The drawing under review shows one solid part. Ordinate dimensions are in mm from its lowest x, y, z. A direction names the side the tool comes from. Round coordinates to 2 decimals unless told otherwise and drop trailing zeros. Write each loop counter-clockwise with the first axis right and the second up, starting at its lowest first coordinate (ties: lowest second). Pieces come first, ordered by that corner, then holes. Notation, with made-up numbers: (-37.5, 71) - (-15.5, 71) arc R22 ccw to (-15.5, 80) - close; hole circle Ø4 at (76, 27.5). An arc over 180 degrees is marked (long way). One line per question, with ' | ' between items. Start each with the question number.
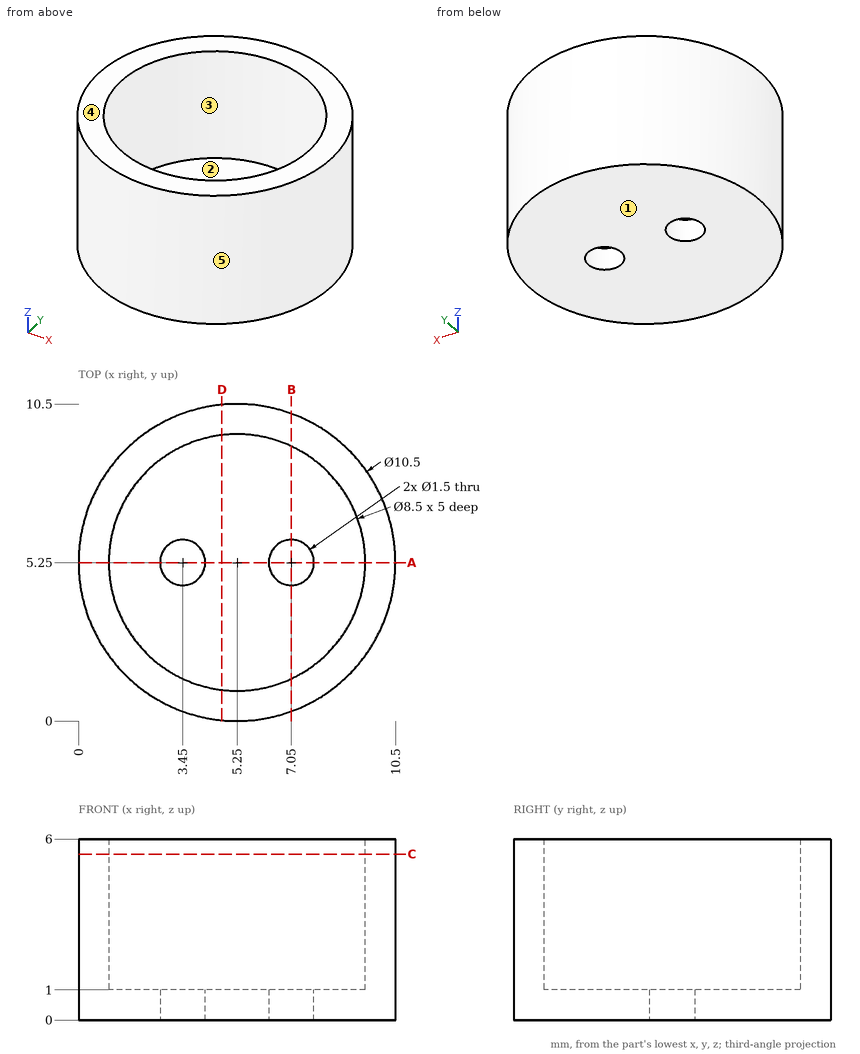
1. Add section B-B, the plane x = 7.05. Write out the cut boundary in (y, z).
2. The part is to be moulded in two halves that separate along Y. For the marked faces 3, 4 and 5, say which applies: pulls with the +Y half, pulls with the -Y half, needs draft (parallel to the pull), parting line crosses it, or undercut.
3. Machinability: for the marked faces 1 and 2, which of the approach directions +Z, -Z, +X, -X, +Y, -Y give a long, thin tool a straight path to every point of the face, cutting with its end or side? Answer none if there is none.
4. Clearance check with flat-ended pins moving along their axes: P1, Ø1.7, axis at x = 7.05, y = 5.25, coming from the +Z side; P2, Ø1.5, axis at x = 7.5, z = 5, coming from the -Y side; P3, Ø3, axis at y = 7, z = 1, coming from the +X side. State where each tip first meets the part, or that it passes through.
5. Add section D-D, the plane x = 4.75. Write out the cut boundary in (y, z), then the cut area to 3 significant figures.
6. Add section A-A, the plane y = 5.25. Write out the cut boundary in (x, z).
7. Wall thickness on line 1 along Y through (x, z) = (5.25, 2.75); line 2 along Z through (x, y) = (5, 4.5); line 3 along Y through (x, z) = (3, 2.3): over which ranges is each line inside the solid? List them lowest first. Write a range as [from, to].
8. Add section C-C, the plane z = 5.5. Write out the cut boundary in (x, y).
Geometry check:
1) outline: (0.32, 0) - (4.5, 0) - (4.5, 1) - (1.4, 1) - (1.4, 6) - (0.32, 6) - close; (6, 0) - (10.18, 0) - (10.18, 6) - (9.1, 6) - (9.1, 1) - (6, 1) - close
2) face 3: undercut | face 4: needs draft | face 5: parting line crosses it
3) face 1: -Z, +X, -X, +Y, -Y | face 2: +Z
4) P1: stops at z = 1 | P2: stops at y = 0.22 | P3: stops at x = 10.49
5) outline: (0.02, 0) - (10.48, 0) - (10.48, 6) - (9.47, 6) - (9.47, 1) - (1.03, 1) - (1.03, 6) - (0.02, 6) - close | area: 20.5 mm2
6) outline: (0, 0) - (2.7, 0) - (2.7, 1) - (1, 1) - (1, 6) - (0, 6) - close; (4.2, 0) - (6.3, 0) - (6.3, 1) - (4.2, 1) - close; (7.8, 0) - (10.5, 0) - (10.5, 6) - (9.5, 6) - (9.5, 1) - (7.8, 1) - close
7) line 1: y = [0, 1], [9.5, 10.5] | line 2: z = [0, 1] | line 3: y = [0.51, 1.64], [8.86, 9.99]
8) outline: circle Ø10.5 at (5.25, 5.25); hole circle Ø8.5 at (5.25, 5.25)
